Check sheet for the drawn part. Datum: minimum x, y, z corner. Units: mm. A direction names the side the tool comes from. Give positions to 0.01 mm unless a question says otherwise; leave off trailing zeros. Loops run counter-clockwise (first coordinate to the right, second up) from the corner with the lowest first, then second, coordinate; pieces in that order, holes last. Notation, with made-up numbers: (2, 18.25) - (9, 18.25) arc R22 cw to (9, 28.25) - close; hole circle Ø4 at (54.25, 68.25). An arc over 180 degrees is marked (long way). Use one line per item in the form item = value.
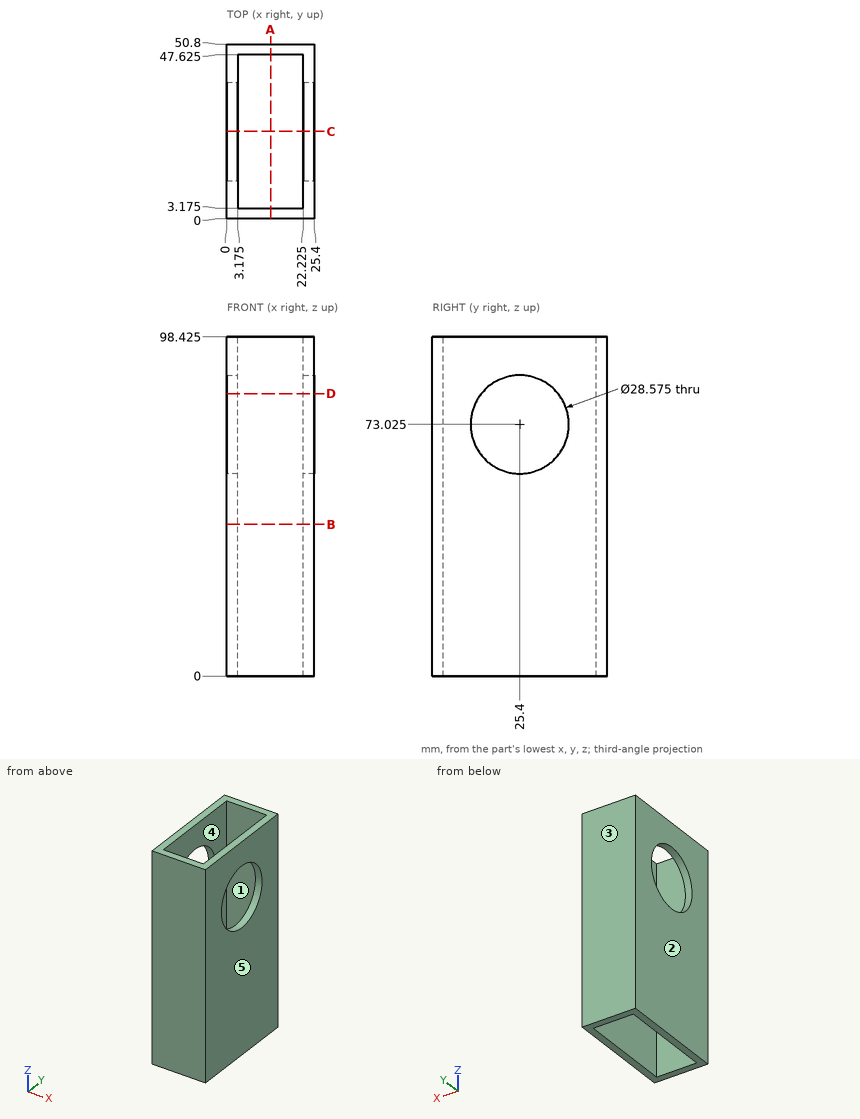
Item 1: Thickness scan on L1, parallel to X at y = 19, z = 18.5 (3 decimals); L2, parallel to Y at x = 13.5, z = 70.5 (3 decimals). Record the ranges inside material, lowest first.
Answer block:
L1 = 0 to 3.175, 22.225 to 25.4
L2 = 0 to 3.175, 47.625 to 50.8
Item 2: Section check A-A on x = 12.75. Record the boundary of the cut face in (y, z) (3 decimals), then the cut area to 3 significant figures.
Answer block:
outline = (0, 0) - (3.175, 0) - (3.175, 98.425) - (0, 98.425) - close; (47.625, 0) - (50.8, 0) - (50.8, 98.425) - (47.625, 98.425) - close
area = 625 mm2
Item 3: Access from +Z, -Z, +X, -X, +Y, -Y to the whole of each face (thin tool, end or side, straight path). Record for the marked faces 4 and 5.
Answer block:
face_4 = +Z, -Z
face_5 = +Z, -Z, +X, +Y, -Y
Item 4: Section check B-B on z = 44. Record the boundary of the cut face in (x, y) (3 decimals), then the cut area to 3 significant figures.
Answer block:
outline = (0, 0) - (25.4, 0) - (25.4, 50.8) - (0, 50.8) - close; hole (3.175, 3.175) - (22.225, 3.175) - (22.225, 47.625) - (3.175, 47.625) - close
area = 444 mm2
Item 5: Section check D-D on z = 82. Record the boundary of the cut face in (x, y) (3 decimals), then the cut area to 3 significant figures.
Answer block:
outline = (0, 0) - (25.4, 0) - (25.4, 14.283) - (22.225, 14.283) - (22.225, 3.175) - (3.175, 3.175) - (3.175, 14.283) - (0, 14.283) - close; (0, 36.517) - (3.175, 36.517) - (3.175, 47.625) - (22.225, 47.625) - (22.225, 36.517) - (25.4, 36.517) - (25.4, 50.8) - (0, 50.8) - close
area = 302 mm2
Item 6: Section check C-C on y = 25.4. Record the boundary of the cut face in (x, z) (1 decimal), then the cut area to 3 significant figures.
Answer block:
outline = (0, 0) - (3.2, 0) - (3.2, 58.7) - (0, 58.7) - close; (0, 87.3) - (3.2, 87.3) - (3.2, 98.4) - (0, 98.4) - close; (22.2, 0) - (25.4, 0) - (25.4, 58.7) - (22.2, 58.7) - close; (22.2, 87.3) - (25.4, 87.3) - (25.4, 98.4) - (22.2, 98.4) - close
area = 444 mm2
Item 7: Mould release check, pull along X, two halves, no side actions. Record for the marked faces 1, 2 and 3: released by +X, released by -X, zero draft, split by the parting line, or undercut.
Answer block:
face_1 = undercut
face_2 = released by -X
face_3 = zero draft
